The listing builds one solid part. Answer for the finished solid, in the listing's coordinates (mm). Face numbers are marked on the shaded views. A direction names the side the tool comes from. Coordinates: 2 decimals unless noted, no trailing zeros. Order: outer loops, then holes, each group sorted by start corner. A loop starts at its lowest first (then second) coordinate and runs counter-clockwise, first axis right, second up. Notation, with made-up numbers: M 5,-33.5 L 35,-33.5 A27 cw 35,-5.5 Z; hole C -8,77.25 d5. An arc over 180 degrees is marked long. One line per item, written item: value. Start each with the question number.
Q1. Determine the mould class of the marked faces 6, 7 and 8 for opening direction X: pulls with the +X half, pulls with the -X half, needs draft (parallel to the pull), parting line crosses it, or undercut.
Q2. The part is cut by section B-B on x = 75. Give the vertices of the cut face in (y, z) (1 decimal).
Q3. Each of these flat-tipped pins is pushed along its axis until it touches: pin 1 Ø8 at (x, z) = (72, -8.5) entering from -Y; pin 2 Ø4 at (x, y) = (78.5, 58) entering from +Z; pin 3 Ø8 at (y, z) = (31, -3) entering from -X. Where does it stop, or does it pass through?
Q4. The part is cut by section D-D on x = 93. Give the vertices of the cut face in (y, z) (3 decimals).
Q5. Straight lines are drawn through the part: line 1 along X through (y, z) = (6, -53.5) (3 decimals); line 2 along Y through (x, z) = (-4.5, 43) (3 decimals); line 3 along Z through (x, y) = (25, 15.5). For each, find the intervals that lie inside material, in ascending order. Write a range as [from, to].
Q6. For the marked faces 1, 2, 3, 4 and 5, determine the directions among +Z, -Z, +X, -X, +Y, -Y from which every point of the face is accessible in a straight line to the end or side of a thin tool.
Q7. The part is cut by section C-C on z = -36. Give the vertices of the cut face in (x, y) (3 decimals).
Q8. The part is cut by section A-A on y = -3.5. Give the vertices of the cut face in (x, z) (3 decimals), then the cut area to 3 significant figures.
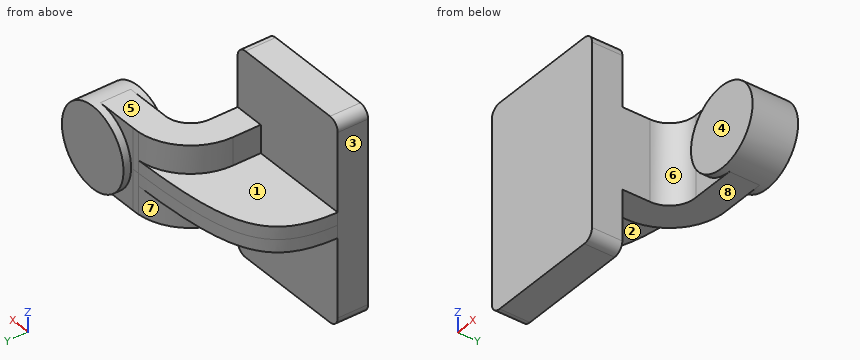
```python
from build123d import *

# Parameters (mm, degrees)
F1_DEPTH = 63.5
F0_W     = 25.4
F0_H     = 19.05
F2_DEPTH = 25.4
F3_DEPTH = 7.9375
F5_R     = 6.35


with BuildPart() as f1:
    # F0 (on Top) → F1 (new body, symmetric)
    with BuildSketch(Plane.XY):
        Polygon((41.275, -9.525), (41.275, 9.525), (22.225, 9.525), (-41.275, 9.525), (-41.275, -9.525), align=None)
    extrude(amount=F1_DEPTH, both=True)

    # F0 (on Top) → F2 (join, symmetric)
    with BuildSketch(Plane.XY):
        with BuildLine():
            Line((22.225, 9.525), (41.275, 9.525))
            Line((41.275, 9.525), (41.275, 27.0309934289))
            ThreePointArc((41.275, 27.0309934289), (46.3478401758, 38.6640913883), (58.3243188197, 42.8625))
            Line((58.3243188197, 42.8625), (60.325, 42.8625))
            Line((60.325, 42.8625), (60.325, 61.9125))
            Line((60.325, 61.9125), (58.8924477992, 61.9125))
            add(Edge.make_bspline(
                [(54.4796435379, 61.8537564061), (55.9299212124, 61.8766562618), (57.4007696655, 61.8961838395), (58.8924477992, 61.9125)],
                knots=[110.8863005517, 110.8863005517, 110.8863005517, 110.8863005517, 113.0396733667, 113.0396733667, 113.0396733667, 113.0396733667], degree=3))
            ThreePointArc((54.4796435379, 61.8537564061), (31.5275701344, 50.7638127469), (22.225, 27.0309934289))
            Line((22.225, 27.0309934289), (22.225, 9.525))
        make_face()
        with Locations((73.025, 52.3875)):
            Rectangle(F0_W, F0_H)
    extrude(amount=F2_DEPTH, both=True)

    # F0 (on Top) → F3 (join, symmetric)
    with BuildSketch(Plane.XY):
        with BuildLine():
            Line((-41.275, 9.525), (22.225, 9.525))
            Line((22.225, 9.525), (22.225, 27.0309934289))
            ThreePointArc((22.225, 27.0309934289), (31.5275701344, 50.7638127469), (54.4796435379, 61.8537564061))
            add(Edge.make_bspline(
                [(-41.275, 9.525), (-40.3356067229, 50.553210625), (-20.2013057937, 60.6745456992), (54.4796435379, 61.8537564061)],
                knots=[0, 0, 0, 0, 110.8863005517, 110.8863005517, 110.8863005517, 110.8863005517], degree=3))
        make_face()
    extrude(amount=F3_DEPTH, both=True)

    # F0 (on Top) → F4 (revolve)
    with BuildSketch(Plane.XY):
        Polygon((85.725, 61.9125), (85.725, 42.8625), (85.725, 38.1), (111.125, 38.1), (111.125, 66.675), (85.725, 66.675), align=None)
    revolve(axis=Axis((85.725, 52.3875, 0), (0, 1, 0)))

    # F5
    f5_edges = [f1.edges().sort_by_distance(p)[0] for p in [
        (-41.275, 0, 63.5),
        (41.275, 0, 63.5),
        (41.275, 0, -63.5),
        (-41.275, 0, -63.5),
    ]]
    fillet(f5_edges, radius=F5_R)


solid = f1.part
```
Output:
1. face 6: undercut
1. face 7: pulls with the -X half
1. face 8: needs draft
2. outline: M 38.1,-23 L 42.9,-23 L 42.9,-25.4 L 61.9,-25.4 L 61.9,-23 L 66.7,-23 L 66.7,23 L 61.9,23 L 61.9,25.4 L 42.9,25.4 L 42.9,23 L 38.1,23 Z
3. pin 1: stops at y = 38.1
3. pin 2: stops at z = 25.4
3. pin 3: stops at x = -39.19
4. outline: M 38.1,-24.336 L 66.675,-24.336 L 66.675,24.336 L 38.1,24.336 Z
5. line 1: x = [-41.275, 41.275]
5. line 2: y = [-9.525, 9.525]
5. line 3: z = [-25.4, 25.4]
6. face 1: +Z, -X, +Y
6. face 2: -Z, -X, +Y
6. face 3: +Z, -Z, -X, +Y, -Y
6. face 4: +Z, -Z, +X, -Y
6. face 5: +Z, +X, -X, +Y
7. outline: M -41.275,-9.525 L 41.275,-9.525 L 41.275,9.525 L -41.275,9.525 Z
8. outline: M -41.275,-57.15 A6.35 ccw -34.925,-63.5 L 34.925,-63.5 A6.35 ccw 41.275,-57.15 L 41.275,57.15 A6.35 ccw 34.925,63.5 L -34.925,63.5 A6.35 ccw -41.275,57.15 Z
8. area: 10,400 mm^2
